Autodesk Inventor part; units mm, degrees
ref_plane "Start Plane" through (0, 0, 0) normal (0, 0, 1) x (1, 0, 0)
ref_plane "End Plane" through (0, 0, 898) normal (0, 0, 1) x (1, 0, 0)
ref_plane "YZ Plane" through (0, 0, 0) normal (1, 0, 0) x (0, 1, 0)
ref_plane "Start Plane" through (0, 0, 0) normal (0, 0, 1) x (1, 0, 0)
ref_plane "End Plane" through (0, 0, 898) normal (0, 0, 1) x (1, 0, 0)
sketch "Sketch" plane through (0, 0, 0) normal (0, 0, 1) x (1, 0, 0)
  line L0 (-20, -16) -> (-20, 16)
  line L1 (-16, 20) -> (16, 20)
  line L2 (20, 16) -> (20, -16)
  line L3 (16, -20) -> (-16, -20)
  arc A0 (-20, -16) -> (-16, -20) centre (-16, -16) ccw
  arc A1 (20, 16) -> (16, 20) centre (16, 16) ccw
  arc A2 (-16, 20) -> (-20, 16) centre (-16, 16) ccw
  arc A3 (16, -20) -> (20, -16) centre (16, -16) ccw
  arc A4 (-16, 18) -> (-18, 16) centre (-16, 16) ccw
  line L4 (-16, 18) -> (16, 18)
  arc A5 (18, 16) -> (16, 18) centre (16, 16) ccw
  line L5 (18, 16) -> (18, -16)
  arc A6 (16, -18) -> (18, -16) centre (16, -16) ccw
  line L6 (16, -18) -> (-16, -18)
  arc A7 (-18, -16) -> (-16, -18) centre (-16, -16) ccw
  line L7 (-18, -16) -> (-18, 16)
  line L8 (0, 29.1598) -> (0, -29.1598) construction
  line L9 (-29.1598, 0) -> (29.1598, 0) construction
  dimension "d7" = 4
  dimension "d9" = 40
  dimension "d11" = 40
  dimension "d12" = 2
  dimension "d15" = 20
  dimension "d16" = 20
extrude "Body" add sketch "Sketch" along normal up to surface (898 mm away) from surface at 0
sketch "Sketch3" plane through (0, 0, 0) normal (0, 0, 1) x (1, 0, 0)
  line L0 (0, 0) -> (10, 0)
ref_plane "Work Plane3" through (0, 0, 0) normal (0, -1, 0) x (1, 0, 0)
sketch "Sketch4" plane through (0, 0, 0) normal (0, -1, 0) x (1, 0, 0)
  line L0 (-2, 0) -> (12, 0)
  line L1 (-2, 898) -> (12, 898)
  dimension "d18" = 898
equation "\"d7\" = G_IR"
equation "\"d9\" = G_W"
equation "\"d11\" = G_H"
equation "\"d12\" = G_T"
equation "\"d15\" = 0.5 * d9"
equation "\"d16\" = 0.5 * d11"
equation "\"d3\" = G_L"
equation "\"G_W\" = 40"
equation "\"G_H\" = 40"
equation "\"G_T\" = 2"
equation "\"G_IR\" = 4"
equation "\"G_L\" = d18"
equation "\"G_OFFSET_START\" = 0"
equation "\"d14\" = G_OFFSET_END + B_L"
equation "\"B_L\" = 938"
properties part number "ISO 4019 - 40x40x2 - 898" material "Steel, Mild"
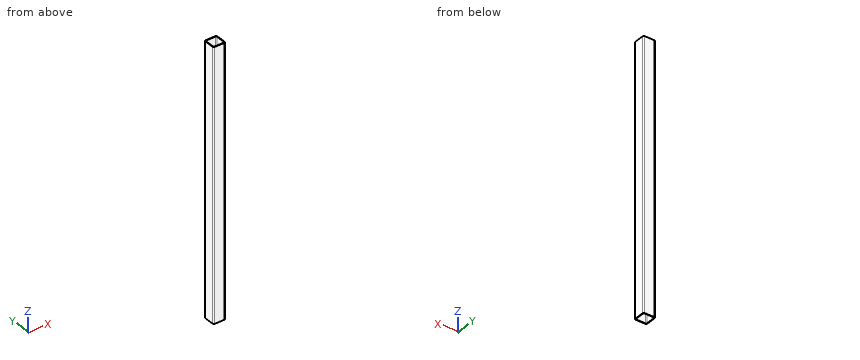
Source: CAD feature listing. Evaluate the final solid. Frame: model axes, mm. Coordinates: 2 decimals unless noted, no trailing zeros. Loops run counter-clockwise (first coordinate to the right, second up) from the corner with the lowest first, then second, coordinate; pieces in that order, holes last. Notation, with made-up numbers: (9, 66.5) -> (22, 66.5) arc R20 cw to (22, 96.5) -> close; hole circle Ø5 at (36, -30.5). An arc over 180 degrees is marked (long way). One line per item, written item: value. Start each with the question number.
Q1. Section query A-A, the plane x = 0.5. Return the cut outline in (y, z).
Q2. Section query C-C, the plane z = 311. Return the cut outline in (x, y), and give its area (3 significant figures).
Q3. Line query: line 1 along X through (y, z) = (16, 152.5); line 2 along X through (y, z) = (16.5, 736). Output: solid intervals per line, ascending.
Results:
1. outline: (-20, 0) -> (-18, 0) -> (-18, 898) -> (-20, 898) -> close; (18, 0) -> (20, 0) -> (20, 898) -> (18, 898) -> close
2. outline: (-20, -16) arc R4 ccw to (-16, -20) -> (16, -20) arc R4 ccw to (20, -16) -> (20, 16) arc R4 ccw to (16, 20) -> (-16, 20) arc R4 ccw to (-20, 16) -> close; hole (-18, -16) arc R2 ccw to (-16, -18) -> (16, -18) arc R2 ccw to (18, -16) -> (18, 16) arc R2 ccw to (16, 18) -> (-16, 18) arc R2 ccw to (-18, 16) -> close
2. area: 294 mm^2
3. line 1: -20 to -18, 18 to 20
3. line 2: -19.97 to -17.94, 17.94 to 19.97
